```python
from build123d import *

# Parameters (mm, degrees)
F0_R     = 50.8
F0_R_2   = 44.45
F1_DEPTH = 54.864
F3_DEPTH = 61.976


# Not quite as in the source:
# - the program builds the solid bodies; features that only make, move or delete a surface that nothing else refers to are left out


with BuildPart() as f1:
    # F0 (on Top) → F1 (new body, symmetric)
    with BuildSketch(Plane.XY):
        Circle(F0_R)
        Circle(F0_R_2, mode=Mode.SUBTRACT)
    extrude(amount=F1_DEPTH, both=True)

    # F0 (on Top) → F3 (join)
    with BuildSketch(Plane.XY):
        Circle(F0_R_2)
    extrude(amount=-F3_DEPTH)


solid = f1.part
```
Input: part model. Units: mm. Frame: model coordinates. A direction names the side the tool comes from. Give positions to 0.01 mm unless a question says otherwise; leave off trailing zeros. Order: outer loops, then holes, each group sorted by start corner. A loop starts at its lowest first (then second) coordinate and runs counter-clockwise, first axis right, second up.
1. Section A-A on x = 0. Return the cut outline in (y, z).
Derived:
outline: (-50.8, -54.86) - (-44.45, -54.86) - (-44.45, -61.98) - (44.45, -61.98) - (44.45, -54.86) - (50.8, -54.86) - (50.8, 54.86) - (44.45, 54.86) - (44.45, 0) - (-44.45, 0) - (-44.45, 54.86) - (-50.8, 54.86) - close
2. Pin query (flat end, axial travel): pin 1 (12 mm diameter, centred on y = 31, z = -27.5, fed in from +X); pin 2 (12 mm diameter, centred on y = 27.5, z = 23.5, fed in from -X); pin 3 (12 mm diameter, centred on x = 14, z = 4, fed in from +Y). Return the tip coordinate at first contact, or that it passes through.
Derived:
pin 1: stops at x = 44.22
pin 2: stops at x = -46.03
pin 3: stops at y = 50.17
3. Material intervals for L1, parallel to Y at x = 0, z = 16; L2, parallel to Z at x = -19, y = 13; L3, parallel to Z at x = 38.5, y = -24.5, sorted ascending.
Derived:
L1: y = -50.8 to -44.45, 44.45 to 50.8
L2: z = -61.98 to 0
L3: z = -54.86 to 54.86
4. Reachability of faces 4 (the cylindrical face through (42.397, 13.352, -58.37)), 5 (the flat face through (-1, 1, 0)), 6 (the flat face through (-1, 1, -61.976)) from +Z, -Z, +X, -X, +Y, -Y: full face, straight path, thin tool, end or side. Return the list, or none.
Derived:
face 4: -Z
face 5: +Z
face 6: -Z, +X, -X, +Y, -Y
5. Section C-C on z = 39.5. Return the cut outline in (x, y), and give its area (3 significant figures).
Derived:
outline: circle Ø101.6 at (0, 0); hole circle Ø88.9 at (0, 0)
area: 1,900 mm2
6. Mould query, pull axis Y, two halves, no side actions, for faces 1 (the cylindrical face through (42.397, 13.352, 27.048)), 2 (the cylindrical face through (-11.012, -49.592, 0.768)), 3 (the flat face through (0, -45, 54.864)). Classes: released by +Y, released by -Y, zero draft, split by the parting line, or undercut.
Derived:
face 1: undercut
face 2: split by the parting line
face 3: zero draft
